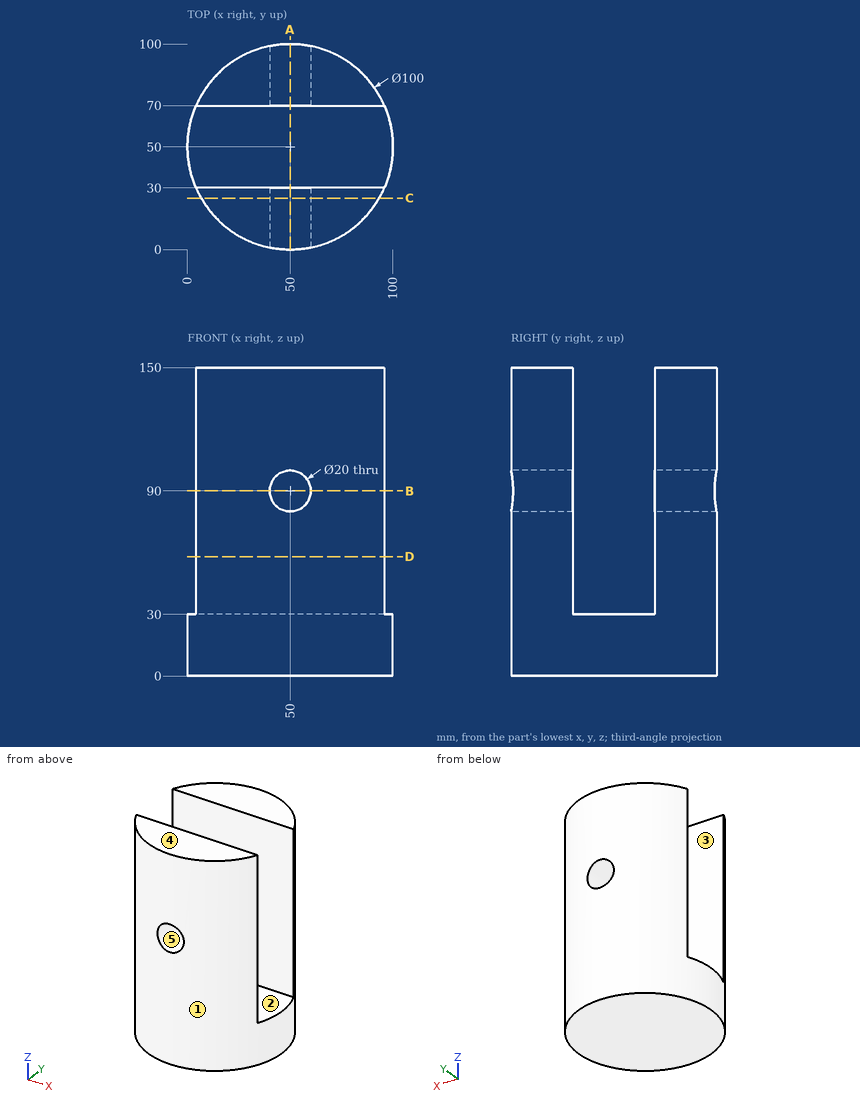
Geometry: see drawing. Coordinates: mm, zero at the bounding-box minimum. A direction names the side the tool comes from. Coordinates: 2 decimals unless noted, no trailing zeros. Order: outer loops, then holes, each group sorted by start corner. A loop starts at its lowest first (then second) coordinate and runs counter-clockwise, first axis right, second up. Notation, with made-up numbers: M 6.25,-17 L 64.25,-17 A18 cw 64.25,13 Z; hole C 7.5,43.5 d9. An arc over 180 degrees is marked long. Write each question's results on one line, items separated by ' | '. Start each with the question number.
1) Section query C-C (y = 25). Return the cut outline in (x, z).
2) Section query D-D (z = 58). Return the cut outline in (x, y).
3) Section query B-B (z = 90). Return the cut outline in (x, y).
4) Section query A-A (x = 50). Return the cut outline in (y, z).
5) Contact query for flat-ended pins moving along their axis: pin 1 Ø1.5 at (x, z) = (13, 87) entering from +Y; pin 2 Ø1.5 at (y, z) = (82, 33.5) entering from -X; pin 3 Ø2 at (x, z) = (42, 107.5) entering from +Y. Output: stop coordinate, or through.
6) Access query for the marked faces 1 and 2. Directions: +Z, -Z, +X, -X, +Y, -Y. A direction counts if a zero-diameter tool reaches every point of the face in a straight line with its end or side. Return the directions, or none.
7) Draft query along Z for the marked faces 3, 4 and 5. Return one class per face: released by +Z, released by -Z, zero draft, split by the parting line, or undercut.
8) Line query: line 1 (Z direction, x = 50, y = 91); line 2 (Y direction, x = 50, z = 64); line 3 (Z direction, x = 76, y = 44). Output: solid intervals per line, ascending. Write a range as from..to.
Answers:
1) outline: M 6.7,0 L 93.3,0 L 93.3,150 L 6.7,150 Z; hole C 50,90 d20
2) outline: M 4.17,30 A50 ccw 95.83,30 Z; M 4.17,70 L 95.83,70 A50 ccw Z
3) outline: M 4.17,30 A50 ccw 40,1.01 L 40,30 Z; M 4.17,70 L 40,70 L 40,98.99 A50 ccw Z; M 60,1.01 A50 ccw 95.83,30 L 60,30 Z; M 60,70 L 95.83,70 A50 ccw 60,98.99 Z
4) outline: M 0,0 L 100,0 L 100,80 L 70,80 L 70,30 L 30,30 L 30,80 L 0,80 Z; M 0,100 L 30,100 L 30,150 L 0,150 Z; M 70,100 L 100,100 L 100,150 L 70,150 Z
5) pin 1: stops at y = 84.44 | pin 2: stops at x = 10.97 | pin 3: stops at y = 99.51
6) face 1: +Z, -Z | face 2: +Z, +X, -X
7) face 3: zero draft | face 4: released by +Z | face 5: undercut
8) line 1: z = 0..80, 100..150 | line 2: y = 0..30, 70..100 | line 3: z = 0..30
